Read the model definition and answer for the solid it produces. Units are mm, in the model's axes. A direction names the side the tool comes from. Coordinates: 2 decimals unless noted, no trailing zeros. Write each loop counter-clockwise with the first axis right and the second up, starting at its lowest first coordinate (ties: lowest second). Pieces come first, ordered by that corner, then holes.
Item 1: Straight lines are drawn through the part: probe 1 along Y at (x, z) = (-232, -438); probe 2 along Z at (x, y) = (-416, -207); probe 3 along Z at (x, y) = (58, -73). For each, find the intervals that lie inside material, in ascending order.
Item 2: This flat-tipped pin is pushed along its axis until it touches: P1, Ø6, axis at x = 386, y = 250.5, coming from the -Z side. Where does it stop, or does it pass through?
Item 3: Section A-A (x = -72.5) is taken. Give the vertices of the cut face in (y, z), then the cut area to 3 significant figures.
Item 4: Section B-B (y = 266) is taken. Give the vertices of the cut face in (x, z), then the cut area to 3 significant figures.
Item 5: Determine the mould class of faces 1 (the face through (-444.5, 298, -695)), 2 (the face through (444.5, -299, -695)), 3 (the face through (-502, 4, -482.6)) for opening direction X: released by +X, released by -X, zero draft, split by the parting line, or undercut.
Item 6: A tool of negligible diameter and unlimited length cuts with its end or side. For faces 4 (the face through (-19.05, 4, -444)), 5 (the face through (-2, -22, -482.6)), 6 (the face through (0, -4, 44)), 7 (the face through (-482, -279.4, -156)), from which of +Z, -Z, +X, -X, +Y, -Y can it reach the whole face along a straight path? Write none if from no direction.
Item 7: Section C-C (z = -182.5) is taken. Give the vertices of the cut face in (x, y), then the cut area to 3 significant figures.
from build123d import *

# Parameters (mm, degrees)
SKETCH_W     = 406.4
SKETCH_H     = 558.8
SKETCH_W_2   = 444.5
PAD_DEPTH    = 88.9
SKETCH002_W  = 76.2
SKETCH002_H  = 38.1
PAD003_DEPTH = 914.4
SKETCH001_W  = 38.1
SKETCH001_H  = 558.8
PAD004_DEPTH = 76.2
SKETCH003_W  = 1041.4
SKETCH003_H  = 635
PAD005_DEPTH = 12.7


with BuildPart() as part:
    # Sketch → Pad (new body)
    with BuildSketch(Plane.XY):
        Polygon((-520.7, 317.5), (-520.7, 279.4), (-444.5, 279.4), (-444.5, -279.4), (-520.7, -279.4), (-520.7, -317.5), (520.7, -317.5), (520.7, 317.5), align=None)
        with Locations((-203.2, 0)):
            Rectangle(SKETCH_W, SKETCH_H, mode=Mode.SUBTRACT)
        with Locations((260.35, 0)):
            Rectangle(SKETCH_W_2, SKETCH_H, mode=Mode.SUBTRACT)
    extrude(amount=PAD_DEPTH)

    # Sketch002 → Pad003 (join)
    with BuildSketch(Plane.XY):
        with Locations((-482.6, 298.45)):
            Rectangle(SKETCH002_W, SKETCH002_H)
        with Locations((482.6, 298.45)):
            Rectangle(SKETCH002_W, SKETCH002_H)
        with Locations((482.6, -298.45)):
            Rectangle(SKETCH002_W, SKETCH002_H)
        with Locations((-482.6, -298.45)):
            Rectangle(SKETCH002_W, SKETCH002_H)
    extrude(amount=-PAD003_DEPTH)

    # Sketch001 → Pad004 (join)
    with BuildSketch(Plane.XY.offset(-406.4)):
        Polygon((-444.5, 279.4), (-19.05, 279.4), (-19.05, -279.4), (-444.5, -279.4), (-444.5, -317.5), (444.5, -317.5), (444.5, -279.4), (19.05, -279.4), (19.05, 279.4), (444.5, 279.4), (444.5, 317.5), (-444.5, 317.5), align=None)
        with Locations((-501.65, 0)):
            Rectangle(SKETCH001_W, SKETCH001_H)
        with Locations((501.65, 0)):
            Rectangle(SKETCH001_W, SKETCH001_H)
    extrude(amount=-PAD004_DEPTH)

    # Sketch003 → Pad005 (join)
    with BuildSketch(Plane.XY.offset(-406.4)):
        Rectangle(SKETCH003_W, SKETCH003_H)
    extrude(amount=PAD005_DEPTH)


solid = part.part
Established:
1. probe 1: y = -317.5 to -279.4, 279.4 to 317.5
1. probe 2: z = -406.4 to -393.7, 0 to 88.9
1. probe 3: z = -406.4 to -393.7
2. P1: stops at z = -406.4
3. outline: (-317.5, -482.6) - (-279.4, -482.6) - (-279.4, -406.4) - (279.4, -406.4) - (279.4, -482.6) - (317.5, -482.6) - (317.5, -393.7) - (-317.5, -393.7) - close; (-317.5, 0) - (-279.4, 0) - (-279.4, 88.9) - (-317.5, 88.9) - close; (279.4, 0) - (317.5, 0) - (317.5, 88.9) - (279.4, 88.9) - close
3. area: 20,600 mm2
4. outline: (-520.7, -482.6) - (-482.6, -482.6) - (-482.6, -406.4) - (-19.05, -406.4) - (-19.05, -482.6) - (19.05, -482.6) - (19.05, -406.4) - (482.6, -406.4) - (482.6, -482.6) - (520.7, -482.6) - (520.7, -393.7) - (-520.7, -393.7) - close; (-444.5, 0) - (-406.4, 0) - (-406.4, 88.9) - (-444.5, 88.9) - close; (0, 0) - (38.1, 0) - (38.1, 88.9) - (0, 88.9) - close; (482.6, 0) - (520.7, 0) - (520.7, 88.9) - (482.6, 88.9) - close
4. area: 32,100 mm2
5. face 1: undercut
5. face 2: undercut
5. face 3: zero draft
6. face 4: -Z
6. face 5: -Z, +Y, -Y
6. face 6: +Z
6. face 7: +Z, -X
7. outline: (-520.7, -317.5) - (-444.5, -317.5) - (-444.5, -279.4) - (-520.7, -279.4) - close; (-520.7, 279.4) - (-444.5, 279.4) - (-444.5, 317.5) - (-520.7, 317.5) - close; (444.5, -317.5) - (520.7, -317.5) - (520.7, -279.4) - (444.5, -279.4) - close; (444.5, 279.4) - (520.7, 279.4) - (520.7, 317.5) - (444.5, 317.5) - close
7. area: 11,600 mm2
